The drawing under review shows one solid part. Ordinate dimensions are in mm from its lowest x, y, z. A direction names the side the tool comes from. Coordinates: 2 decimals unless noted, no trailing zeros. Order: outer loops, then holes, each group sorted by start corner. A loop starts at its lowest first (then second) coordinate and runs counter-clockwise, first axis right, second up. Notation, with made-up numbers: (7.5, -4) - (39.5, -4) arc R18 ccw to (39.5, 18) - close; hole circle Ø2 at (12, 51.5). An arc over 180 degrees is marked (long way). Answer in a Markdown table with one row per item.
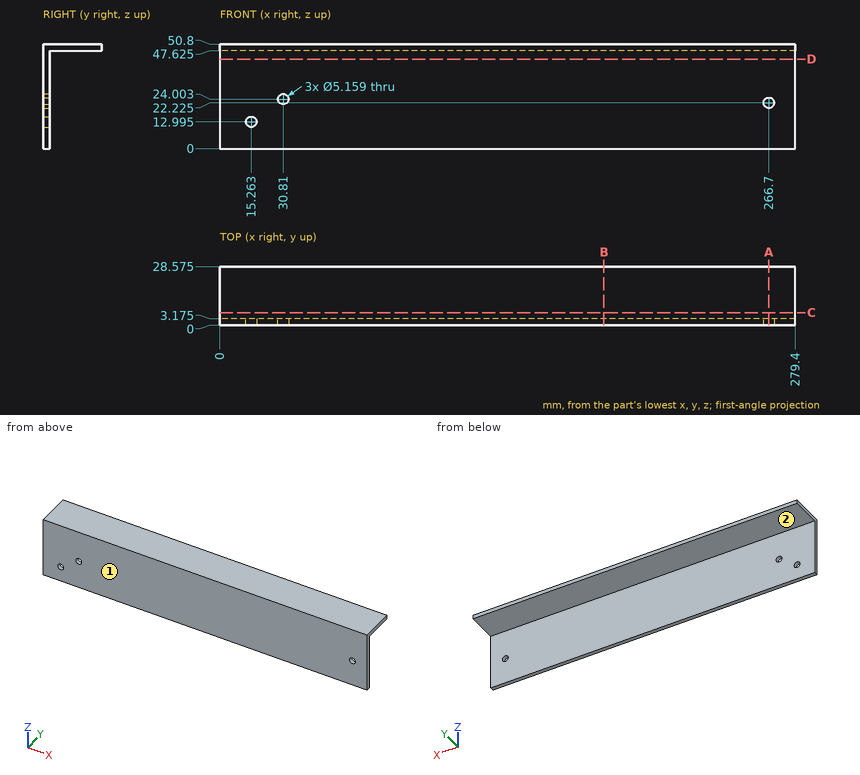
Item 1: We need section C-C, the plane y = 6.25. Write out the cut boundary in (x, z) (1 decimal).
Check values:
| item | result |
|---|---|
| outline | (0, 47.6) - (279.4, 47.6) - (279.4, 50.8) - (0, 50.8) - close |
Item 2: Clearance check with flat-ended pins moving along their axes: pin 1 Ø14.5 at (x, z) = (117, 30) entering from +Y (3 decimals); pin 2 Ø4 at (x, y) = (249.5, 13.5) entering from -Z (3 decimals). State where each tip first meets the part, or that it passes through.
Check values:
| item | result |
|---|---|
| pin 1 | y = 3.175 |
| pin 2 | z = 47.625 |
Item 3: We need section B-B, the plane x = 186.5. Write out the cut boundary in (y, z) (1 decimal), then the cut area to 3 significant figures.
Check values:
| item | result |
|---|---|
| outline | (0, 0) - (3.2, 0) - (3.2, 47.6) - (28.6, 47.6) - (28.6, 50.8) - (0, 50.8) - close |
| area | 242 mm^2 |
Item 4: We need section A-A, the plane x = 266.7. Write out the cut boundary in (y, z) (1 decimal).
Check values:
| item | result |
|---|---|
| outline | (0, 0) - (3.2, 0) - (3.2, 19.6) - (0, 19.6) - close; (0, 24.8) - (3.2, 24.8) - (3.2, 47.6) - (28.6, 47.6) - (28.6, 50.8) - (0, 50.8) - close |
Item 5: To check wall thickness, follow line 1 (Z direction, x = 266.7, y = 1.6) (1 decimal); line 2 (Y direction, x = 152, z = 40) (1 decimal); line 3 (Z direction, x = 74.5, y = 26.75) (1 decimal). State the ranges of each line that lie inside material, in increasing order. Write a range as from..to.
Check values:
| item | result |
|---|---|
| line 1 | 0..19.6, 24.8..50.8 |
| line 2 | 0..3.2 |
| line 3 | 47.6..50.8 |
Item 6: We need section D-D, the plane z = 43.5. Write out the cut boundary in (x, y) (1 decimal).
Check values:
| item | result |
|---|---|
| outline | (0, 0) - (279.4, 0) - (279.4, 3.2) - (0, 3.2) - close |
Item 7: Tool access review of the marked faces 1 and 2: name each direction out of +Z, -Z, +X, -X, +Y, -Y from which nothing blocks a thin tool from reaching the whole face with its end or side.
Check values:
| item | result |
|---|---|
| face 1 | +Z, -Z, +X, -X, -Y |
| face 2 | -Z, +X, -X, +Y |
